Source: CAD feature listing. Evaluate the final solid. Frame: model axes, mm. A direction names the side the tool comes from. Give positions to 0.01 mm unless a question says otherwise; leave off trailing zeros. Write each loop counter-clockwise with the first axis right and the second up, starting at its lowest first coordinate (ties: lowest second). Pieces come first, ordered by that corner, then holes.
```python
from build123d import *

# Parameters (mm, degrees)
SKETCH_1_W          = 77
SKETCH_1_H          = 61
EXTRUDE_1_DEPTH     = 108.5
SKETCH_2_W          = 77
SKETCH_2_H          = 77
CUT_EXTRUDE_1_DEPTH = 10
SKETCH_3_W          = 85
SKETCH_3_H          = 4
EXTRUDE_2_DEPTH     = 18


with BuildPart() as part:
    # 草图1 → 凸台-拉伸1 (new body)
    with BuildSketch(Plane.XY):
        with Locations((38.5, 30.5)):
            Rectangle(SKETCH_1_W, SKETCH_1_H)
    extrude(amount=EXTRUDE_1_DEPTH)

    # 草图2 → 切除-拉伸1 (cut)
    with BuildSketch(Plane(origin=(0, 61, 0), x_dir=(1, 0, 0), z_dir=(0, 1, 0))):
        with Locations((38.5, -70)):
            Rectangle(SKETCH_2_W, SKETCH_2_H)
    extrude(amount=-CUT_EXTRUDE_1_DEPTH, mode=Mode.SUBTRACT)

    # 草图3 → 凸台-拉伸2 (add)
    with BuildSketch(Plane(origin=(0, 21.5, 0), x_dir=(-1, 0, 0), z_dir=(0, -1, 0))):
        with Locations((-38.5, -10)):
            Rectangle(SKETCH_3_W, SKETCH_3_H)
    extrude(amount=-EXTRUDE_2_DEPTH)


solid = part.part
```
1. Cut plane A-A, the plane y = 36. Return the cut outline in (x, z), then the cut area to 3 significant figures.
2. Cut plane D-D, the plane y = 46.5. Return the cut outline in (x, z), then the cut area to 3 significant figures.
3. Line query: L1, parallel to X at y = 17, z = 49; L2, parallel to Y at x = 33, z = 85.5; L3, parallel to Z at x = 11, y = 58. Output: solid intervals per line, ascending.
4. Cut plane B-B, the plane z = 29. Return the cut outline in (x, y), then the cut area to 3 significant figures.
5. Cut plane C-C, the plane x = 74.5. Return the cut outline in (y, z), then the cut area to 3 significant figures.
6. Contact query for flat-ended pins moving along their axis: P1, Ø23, axis at x = 55.5, z = 87, coming from the +Y side; P2, Ø10, axis at y = 37.5, z = 51.5, coming from the +X side; P3, Ø1, axis at y = 21, z = 64.5, coming from the -X side. Output: stop coordinate, or through.
7. Access query for faces 1 (the flat face through (79, 30, 8)), 2 (the flat face through (79, 21.5, 10)), 3 (the flat face through (38, 56, 31.5)), 4 (the flat face through (-2, 21.5, 10)), 5 (the flat face through (-2, 39.5, 10)). Directions: +Z, -Z, +X, -X, +Y, -Y. A direction counts if a zero-diameter tool reaches every point of the face in a straight line with its end or side. Return the directions, or none.
Response values:
1. outline: (-4, 8) - (0, 8) - (0, 0) - (77, 0) - (77, 8) - (81, 8) - (81, 12) - (77, 12) - (77, 108.5) - (0, 108.5) - (0, 12) - (-4, 12) - close
1. area: 8,390 mm2
2. outline: (0, 0) - (77, 0) - (77, 108.5) - (0, 108.5) - close
2. area: 8,350 mm2
3. L1: x = 0 to 77
3. L2: y = 0 to 51
3. L3: z = 0 to 31.5
4. outline: (0, 0) - (77, 0) - (77, 61) - (0, 61) - close
4. area: 4,700 mm2
5. outline: (0, 0) - (61, 0) - (61, 31.5) - (51, 31.5) - (51, 108.5) - (0, 108.5) - close
5. area: 5,850 mm2
6. P1: stops at y = 51
6. P2: stops at x = 77
6. P3: stops at x = 0
7. face 1: -Z, +X, +Y, -Y
7. face 2: +Z, -Z, +X, -Y
7. face 3: +Z, +X, -X, +Y
7. face 4: +Z, -Z, -X, -Y
7. face 5: +Z, -Z, -X, +Y
